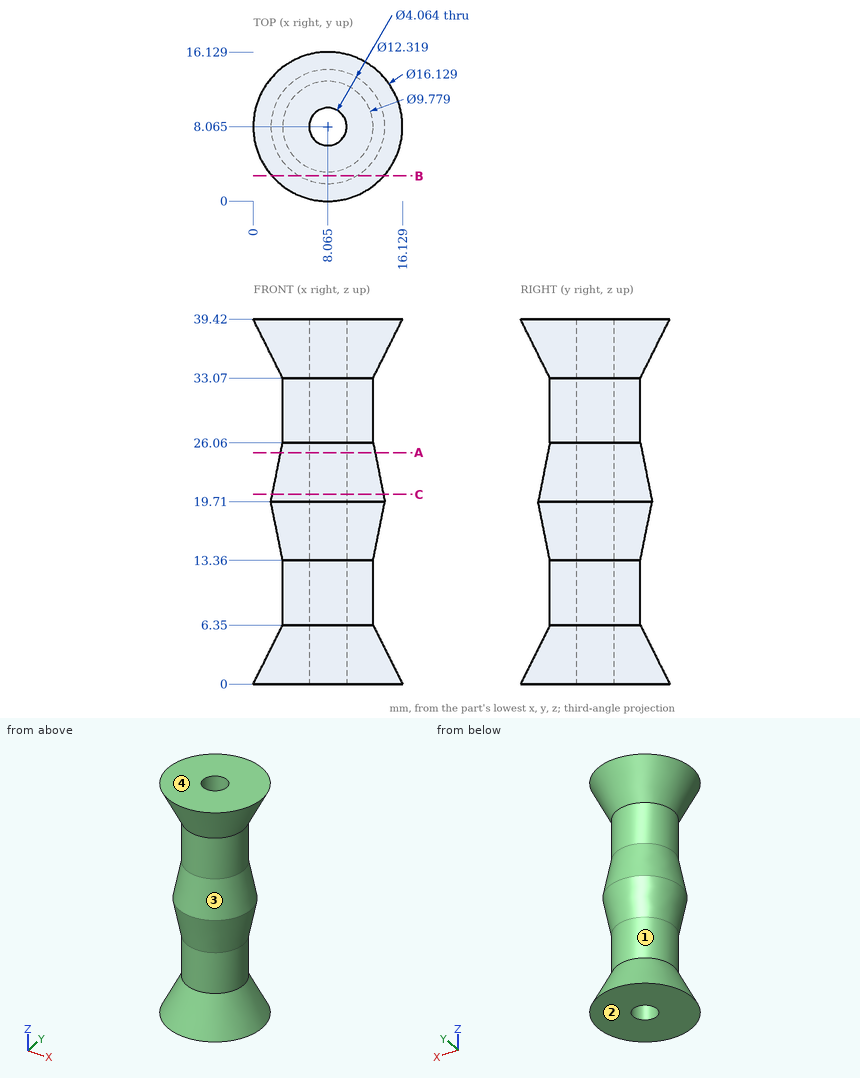
Geometry: see drawing. Coordinates: mm, zero at the bounding-box minimum. Round coordinates to 2 decimals unless told otherwise and drop trailing zeros. Write each loop counter-clockwise with the first axis right and the second up, starting at its lowest first coordinate (ties: lowest second). Pieces come first, ordered by that corner, then holes. Notation, with made-up numbers: M 72,27.25 L 109,27.25 A19 cw 109,55.25 Z; hole C 7.5,-24 d5. An arc over 180 degrees is marked long. Answer in a Markdown table with one row per item. Add a question column.
(1) Cut plane A-A, the plane z = 25. Return the cut outline in (x, y) (1 decimal).
(2) Cut plane B-B, the plane y = 2.75. Give the number of separate pieces and of enclosed holes in the cut face, then the cut area to 3 significant figures.
(3) Ray query, L1, parallel to Z at x = 1.5, y = 5.5 (1 decimal); L2, parallel to Y at x = 7.25, z = 29.5 (1 decimal); L3, parallel to X at y = 7, z = 15 (1 decimal). Return the intervals inside material, ascending.
(4) Contact query for flat-ended pins moving along their axis: pin 1 (6 mm diameter, centred on y = 10, z = 8.5, fed in from +X); pin 2 (2 mm diameter, centred on x = 9, z = 14, fed in from +Y); pin 3 (1 mm diameter, centred on y = 6.5, z = 24, fed in from +X). Output: stop coordinate, or through.
(5) Cut plane C-C, the plane z = 20.5. Return the cut outline in (x, y) (1 decimal), then the cut area to 3 significant figures.
(6) Draft query along Z for the marked faces 1, 2, 3 and 4. Return one class per face: pulls with the +Z half, pulls with the -Z half, needs draft (parallel to the pull), parting line crosses it, or undercut.
Established:
| question | item | result |
|---|---|---|
| 1 | outline | C 8.1,8.1 d10.2; hole C 8.1,8.1 d4.1 |
| 2 | separate pieces | 3 |
| 2 | enclosed holes | 0 |
| 2 | area | 120 mm² |
| 3 | L1 | 0 to 2, 37.4 to 39.4 |
| 3 | L2 | 3.2 to 6.2, 9.9 to 12.9 |
| 3 | L3 | 3 to 6.3, 9.8 to 13.2 |
| 4 | pin 1 | x = 13.21 |
| 4 | pin 2 | y = 13.24 |
| 4 | pin 3 | x = 13.3 |
| 5 | outline | C 8.1,8.1 d12; hole C 8.1,8.1 d4.1 |
| 5 | area | 100 mm² |
| 6 | face 1 | undercut |
| 6 | face 2 | pulls with the -Z half |
| 6 | face 3 | undercut |
| 6 | face 4 | pulls with the +Z half |
